For this review, take the finished solid that the model builds, in its own axes (mm). A direction names the side the tool comes from. Round coordinates to 2 decimals unless told otherwise and drop trailing zeros. Write each loop counter-clockwise with the first axis right and the second up, starting at its lowest first coordinate (ties: lowest second). Pieces come first, ordered by that corner, then holes. Notation, with made-up numbers: (30.5, 79.25) - (35.5, 79.25) arc R14 cw to (35.5, 102.25) - close; hole circle Ø3 at (26.5, 14). An arc over 180 degrees is marked (long way). One line per item, written item: value. Start each with the question number.
Q1. Mouldability with a two-part tool opening along Y and no side actions: class faces 4 (the face through (-46, 183, 1)), 5 (the face through (-49.44, 160.536, 22.959)), 6 (the face through (-68.247, 139.605, 22.643)) as +Y half, -Y half, draft (parallel to the pull), parting line (faces both ways), or undercut.
Q2. Add section C-C on y = 201. Give the number of separate pieces and of enclosed holes in the cut face, and give its area (3 significant figures).
Q3. For probe 1 along Z at (x, y) = (-65, 136); probe 2 along Z at (x, y) = (-49, 208); probe 3 along Z at (x, y) = (-47, 179), list the stretches that pass through material, from the lowest coordinate up.
Q4. Clearance check with flat-ended pins moving along their axes: pin 1 Ø3 at (y, z) = (220, 29) entering from +X; pin 2 Ø9 at (x, z) = (-61.5, 5) entering from +Y; pin 3 Ø3 at (y, z) = (157.5, -7.5) entering from -X. State where each tip first meets the part, or that it passes through.
Q5. Add section A-A on x = -65. Write out the cut boundary in (y, z), and give its area (3 significant figures).
Q6. Add section B-B on z = -12. Write out the cut boundary in (x, y), and give its area (3 significant figures).
Q7. Tool access review of faces 1 (the face through (-44.5, 212, 0.5)), 2 (the face through (56, 179, 1)), 3 (the face through (-52, 205, -20)): name each direction out of +Z, -Z, +X, -X, +Y, -Y from which nothing blocks a thin tool from reaching the whole face with its end or side.
```python
from build123d import *

# Parameters (mm, degrees)
PAD013_DEPTH            = 39
HOLE004_D               = 5.8
HOLE004_DEPTH           = 50
HOLE004_CBORE_D         = 9.5
HOLE004_CBORE_DEPTH     = 7
HOLE004_TIPS_R          = 2.9
CHAMFER003_SIZE         = 1
SKETCH021_R             = 3.25
POCKET003_DEPTH         = 408.975618
BODY005_PLACEMENT_ANGLE = 270


with BuildPart() as part:
    # Sketch019 → Pad013 (new body, symmetric)
    with BuildSketch(Plane.XZ):
        with BuildLine():
            ThreePointArc((-39.987498, -1), (40, 0), (-39.987498, 1))
            Line((-56, 1), (-39.987498, 1))
            Line((-56, 1), (-56, 28))
            Line((-56, 28), (-43.817805, 28))
            ThreePointArc((43.817805, 28), (0, 52), (-43.817805, 28))
            Line((43.817805, 28), (56, 28))
            Line((56, 28), (56, -37))
            Line((74, -37), (56, -37))
            Line((74, -52), (74, -37))
            Line((-74, -52), (74, -52))
            Line((-74, -37), (-74, -52))
            Line((-56, -37), (-74, -37))
            Line((-56, -37), (-56, -1))
            Line((-39.987498, -1), (-56, -1))
        make_face()
    extrude(amount=PAD013_DEPTH, both=True)

    # Hole004
    with Locations(Plane(origin=(0, 0, 28), x_dir=(-1, 0, 0), z_dir=(0, 0, 1))):
        with Locations((49.5, 22.5), (49.5, 0), (49.5, -22.5)):
            CounterBoreHole(HOLE004_D / 2, HOLE004_CBORE_D / 2, HOLE004_CBORE_DEPTH, depth=HOLE004_DEPTH)

    # Hole004 tips → Hole004 tip 1 section 0
    with BuildSketch(Plane(origin=(0, 0, -22), x_dir=(-1, 0, 0), z_dir=(0, 0, 1)), mode=Mode.PRIVATE) as hole004_tip_1_s0:
        with Locations((49.5, 22.5)):
            Circle(HOLE004_TIPS_R)
    loft([hole004_tip_1_s0.sketch, Vertex(-49.5, -22.5, -23.742496)], mode=Mode.SUBTRACT)

    # Hole004 tips → Hole004 tip 2 section 0
    with BuildSketch(Plane(origin=(0, 0, -22), x_dir=(-1, 0, 0), z_dir=(0, 0, 1)), mode=Mode.PRIVATE) as hole004_tip_2_s0:
        with Locations((49.5, 0)):
            Circle(HOLE004_TIPS_R)
    loft([hole004_tip_2_s0.sketch, Vertex(-49.5, 0, -23.742496)], mode=Mode.SUBTRACT)

    # Hole004 tips → Hole004 tip 3 section 0
    with BuildSketch(Plane(origin=(0, 0, -22), x_dir=(-1, 0, 0), z_dir=(0, 0, 1)), mode=Mode.PRIVATE) as hole004_tip_3_s0:
        with Locations((49.5, -22.5)):
            Circle(HOLE004_TIPS_R)
    loft([hole004_tip_3_s0.sketch, Vertex(-49.5, 22.5, -23.742496)], mode=Mode.SUBTRACT)

    # Chamfer003
    chamfer003_edges = [part.edges().sort_by_distance(p)[0] for p in [
        (40, 39, 0),
        (0, 39, 52),
        (-49.908902, 39, 28),
        (-56, 0, 28),
        (49.908902, 39, 28),
        (56, 0, 28),
        (-56, 39, 14.5),
        (-56, 39, -19),
        (-65, 39, -37),
        (-74, 39, -44.5),
        (0, 39, -52),
        (74, 39, -44.5),
        (65, 39, -37),
        (56, 39, -4.5),
        (40, -39, 0),
        (0, -39, 52),
        (-49.908902, -39, 28),
        (49.908902, -39, 28),
        (56, -39, -4.5),
        (65, -39, -37),
        (74, -39, -44.5),
        (0, -39, -52),
        (-74, -39, -44.5),
        (-65, -39, -37),
        (-56, -39, -19),
        (-56, -39, 14.5),
        (-74, 0, -52),
        (74, 0, -52),
    ]]
    chamfer(chamfer003_edges, length=CHAMFER003_SIZE)

    # Sketch021 (on Face54 of Chamfer003) → Pocket003 (cut, through all)
    with BuildSketch(Plane(origin=(0, 0, -37), x_dir=(-1, 0, 0), z_dir=(0, 0, 1))):
        with Locations((-65, 22.5)):
            Circle(SKETCH021_R)
        with Locations((-65, -22.5)):
            Circle(SKETCH021_R)
    pocket003 = extrude(amount=-POCKET003_DEPTH, mode=Mode.SUBTRACT)

    # Mirrored002: Pocket003 across YZ
    add(pocket003.mirror(Plane.YZ), mode=Mode.SUBTRACT)


with BuildPart() as part_1:
    # Body005 placement: moved
    add(part.part.moved(Location((0, 184, 0))).rotate(Axis((0, 184, 0), (1, 0, 0)), BODY005_PLACEMENT_ANGLE))


solid = part_1.part
```
Result set:
1. face 4: undercut
1. face 5: +Y half
1. face 6: draft
2. separate pieces: 2
2. enclosed holes: 3
2. area: 3,000 mm^2
3. probe 1: z = -39 to -25.75, -19.25 to 19.25, 25.75 to 39
3. probe 2: z = -39 to -27.22, -17.78 to -4.72, 4.72 to 17.78, 27.22 to 39
3. probe 3: z = -39 to -23.97, -21.03 to -1.47, 1.47 to 21.03, 23.97 to 39
4. pin 1: stops at x = 38.91
4. pin 2: stops at y = 147
4. pin 3: stops at x = -56
5. outline: (132, -38) - (133, -39) - (146, -39) - (147, -38) - (147, -25.75) - (132, -25.75) - close; (132, -19.25) - (147, -19.25) - (147, 19.25) - (132, 19.25) - close; (132, 25.75) - (147, 25.75) - (147, 38) - (146, 39) - (133, 39) - (132, 38) - close
5. area: 973 mm^2
6. outline: (-74, 133) - (-73, 132) - (73, 132) - (74, 133) - (74, 147) - (56, 147) - (56, 211) - (55, 212) - (43.82, 212) arc R52 ccw to (-43.82, 212) - (-55, 212) - (-56, 211) - (-56, 185) - (-39.99, 185) arc R40 cw (long way) to (-39.99, 183) - (-56, 183) - (-56, 147) - (-74, 147) - close
6. area: 5,920 mm^2
7. face 1: +Z, -Z, -X, +Y
7. face 2: +Z, -Z, +X, +Y
7. face 3: +Y
